Input: dimensioned drawing with shaded views. Units: mm. Origin: part minimum x, y, z. A direction names the side the tool comes from. Give positions to 0.01 mm unless a question says otherwise; leave off trailing zeros. Write each loop counter-clockwise with the first axis right and the second up, starting at its lowest first coordinate (ties: lowest second). Pieces come first, ordered by that corner, then holes. Notation, with made-up numbers: (7, -33.75) -> (56, -33.75) arc R16 cw to (56, -15.75) -> close; hole circle Ø4 at (25.5, 70). An arc over 180 degrees is marked (long way). Answer as a JSON object with one key per item and string values.
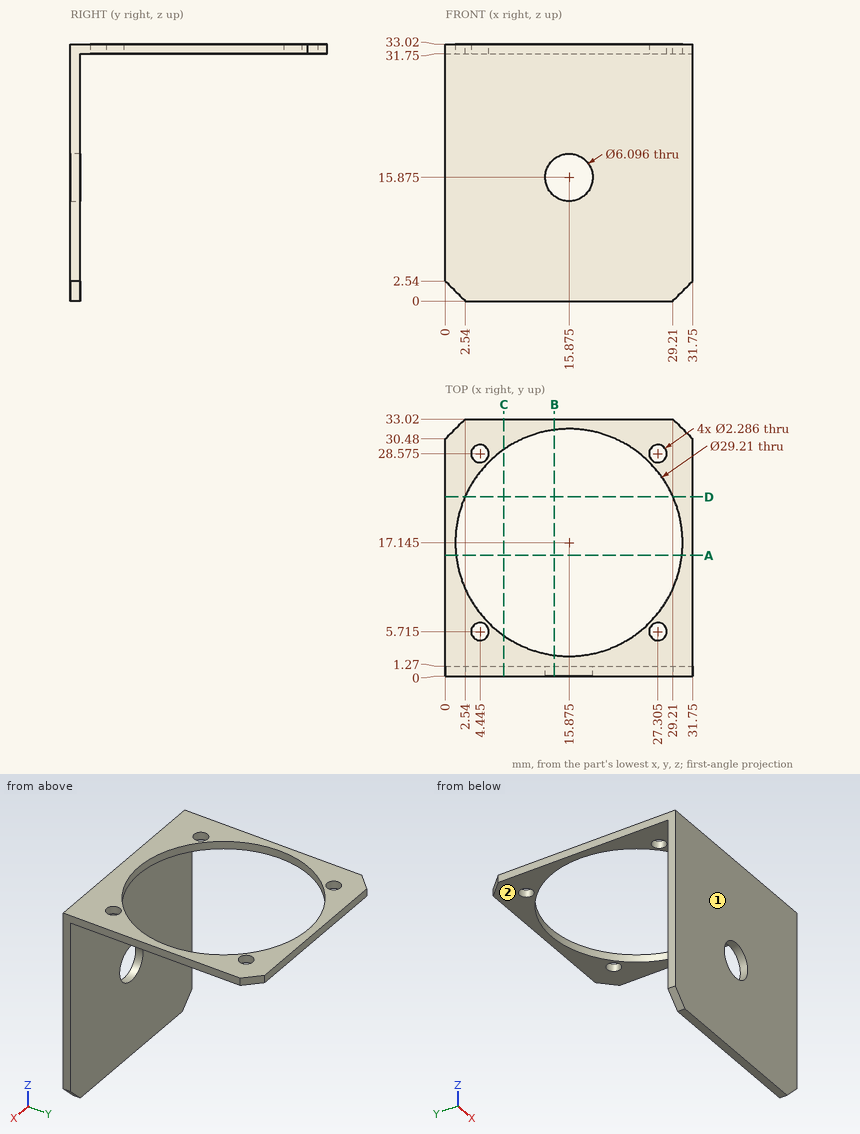
Q1. Cut plane D-D (y = 23). Return the cut outline in (x, z).
Values:
{"outline": "(0, 31.75) -> (2.49, 31.75) -> (2.49, 33.02) -> (0, 33.02) -> close; (29.26, 31.75) -> (31.75, 31.75) -> (31.75, 33.02) -> (29.26, 33.02) -> close"}
Q2. Set-up query: the marked faces 1 and 2. Return all of +Z, -Z, +X, -X, +Y, -Y with unobstructed straight access to the full face (end or side cutting, diameter ignored); none if empty.
Values:
{"face 1": "+Z, -Z, +X, -X, -Y", "face 2": "-Z, +X, -X, +Y"}
Q3. Material intervals for L1, parallel to Y at x = 20, z = 22.5; L2, parallel to Z at x = 27, y = 3, sorted ascending. Write a range as from..to.
Values:
{"L1": "0..1.27", "L2": "31.75..33.02"}
Q4. Cut plane B-B (x = 14). Return the cut outline in (y, z).
Values:
{"outline": "(0, 0) -> (1.27, 0) -> (1.27, 13.47) -> (0, 13.47) -> close; (0, 18.28) -> (1.27, 18.28) -> (1.27, 31.75) -> (2.66, 31.75) -> (2.66, 33.02) -> (0, 33.02) -> close; (31.63, 31.75) -> (33.02, 31.75) -> (33.02, 33.02) -> (31.63, 33.02) -> close"}
Q5. Cut plane A-A (y = 15.5). Return the cut outline in (x, z), and give its area (3 significant figures).
Values:
{"outline": "(0, 31.75) -> (1.36, 31.75) -> (1.36, 33.02) -> (0, 33.02) -> close; (30.39, 31.75) -> (31.75, 31.75) -> (31.75, 33.02) -> (30.39, 33.02) -> close", "area": "3.46 mm²"}
Q6. First-contact query: P1, Ø9.5, axis at x = 21.5, z = 12, coming from the +Y side; P2, Ø3, axis at x = 4.445, y = 5.715, coming from the -Z side. Flat tips, straight axial feed; report the tip coordinate or a pass-through.
Values:
{"P1": "y = 1.27", "P2": "z = 31.75"}
Q7. Cut plane C-C (x = 7.5). Return the cut outline in (y, z).
Values:
{"outline": "(0, 0) -> (1.27, 0) -> (1.27, 31.75) -> (5.18, 31.75) -> (5.18, 33.02) -> (0, 33.02) -> close; (29.11, 31.75) -> (33.02, 31.75) -> (33.02, 33.02) -> (29.11, 33.02) -> close"}
